```python
from build123d import *

# Parameters (mm, degrees)
F1_DEPTH = 2


with BuildPart() as f1:
    # F0 (on Top) → F1 (new body)
    with BuildSketch(Plane.XY):
        with BuildLine():
            Line((-4.25, -12.868576), (-4.25, 0))
            Line((-4.25, 0), (-6.25, 0))
            Line((-6.25, 0), (-6.25, -1))
            Line((-6.25, -1), (-5.018, -1))
            Line((-5.018, -1), (-5.018, -13.788901))
            ThreePointArc((-5.018, -13.788901), (0, -17.016697), (5.018, -13.788901))
            Line((5.018, -13.788901), (5.018, -1))
            Line((5.018, -1), (6.25, -1))
            Line((6.25, -1), (6.25, 0))
            Line((6.25, 0), (4.25, 0))
            Line((4.25, 0), (4.25, -12.868576))
            Line((4.25, -12.868576), (-4.25, -12.868576))
        make_face()
    extrude(amount=F1_DEPTH)


solid = f1.part
```
Check sheet for the modelled part. Datum: model origin and axes. Units: mm. A direction names the side the tool comes from. Give positions to 0.01 mm unless a question says otherwise; leave off trailing zeros. Order: outer loops, then holes, each group sorted by start corner. A loop starts at its lowest first (then second) coordinate and runs counter-clockwise, first axis right, second up. Notation, with made-up numbers: (35.5, 37.5) -> (54.5, 37.5) arc R21 cw to (54.5, 43.5) -> close; hole circle Ø3 at (-6, 4.25). An arc over 180 degrees is marked (long way). Return JSON: item names as keys, results as strings.
1. Cross-section at C-C, the plane x = 4. Record the cut outline in (y, z), plus the area to 3 significant figures.
From the geometry:
{"outline": "(-15.3, 0) -> (-12.87, 0) -> (-12.87, 2) -> (-15.3, 2) -> close", "area": "4.86 mm^2"}
2. Material ranges on probe 1 along X at (y, z) = (-2.75, 0.95); probe 2 along Y at (x, z) = (0.25, 1.1); probe 3 along X at (y, z) = (-13, 0.9), recorded low to high. Write a range as [from, to].
From the geometry:
{"probe 1": "[-5.02, -4.25], [4.25, 5.02]", "probe 2": "[-17.01, -12.87]", "probe 3": "[-5.02, 5.02]"}
3. Go/stop test with flat-tipped pins: P1, Ø0.6, axis at x = -6, z = 1, coming from the -Y side; P2, Ø0.6, axis at y = -9, z = 0.5, coming from the -X side; P3, Ø4, axis at x = 3.5, y = -8, coming from the +Z side; P4, Ø1, axis at y = -5.5, z = 0.5, coming from the +X side. Record where each tip stops, or that it passes through.
From the geometry:
{"P1": "y = -1", "P2": "x = -5.02", "P3": "z = 2", "P4": "x = 5.02"}
4. Cross-section at B-B, the plane z = 1.35. Record the cut outline in (x, y).
From the geometry:
{"outline": "(-6.25, -1) -> (-5.02, -1) -> (-5.02, -13.79) arc R5.51 ccw to (5.02, -13.79) -> (5.02, -1) -> (6.25, -1) -> (6.25, 0) -> (4.25, 0) -> (4.25, -12.87) -> (-4.25, -12.87) -> (-4.25, 0) -> (-6.25, 0) -> close"}
5. Set-up check for faces 5 (the flat face through (6, -1, 1)), 6 (the flat face through (0, -14, 0)), 7 (the flat face through (-4.25, -7, 1)), 8 (the flat face through (-5.018, -7, 1)): record each of +Z, -Z, +X, -X, +Y, -Y from which the full face is reachable in a straight line by a thin tool's end or side.
From the geometry:
{"face 5": "+Z, -Z, +X, -Y", "face 6": "-Z, +X, -X, +Y, -Y", "face 7": "+Z, -Z, +Y", "face 8": "+Z, -Z, -X, -Y"}
6. Cross-section at A-A, the plane y = -2.5. Record the cut outline in (x, z).
From the geometry:
{"outline": "(-5.02, 0) -> (-4.25, 0) -> (-4.25, 2) -> (-5.02, 2) -> close; (4.25, 0) -> (5.02, 0) -> (5.02, 2) -> (4.25, 2) -> close"}
7. Mould release check, pull along X, two halves, no side actions. Record for faces 1 (the flat face through (4.25, -6, 1)), 2 (the flat face through (0, -12.869, 1)), 3 (the flat face through (6.25, -0.5, 1)), 4 (the flat face through (-6, -1, 1)): +X half, -X half, draft (parallel to the pull), parting line (faces both ways), or undercut.
From the geometry:
{"face 1": "undercut", "face 2": "undercut", "face 3": "+X half", "face 4": "draft"}
8. Cross-section at D-D, the plane y = -13.25. Record the cut outline in (x, z), plus the area to 3 significant figures.
From the geometry:
{"outline": "(-5.02, 0) -> (5.02, 0) -> (5.02, 2) -> (-5.02, 2) -> close", "area": "20.1 mm^2"}
